The model under review builds one solid part; all positions refer to its coordinate system, in mm. A direction names the side the tool comes from. Give positions to 0.01 mm unless a question says otherwise; leave off trailing zeros. Loops run counter-clockwise (first coordinate to the right, second up) from the corner with the lowest first, then second, coordinate; pieces in that order, holes last. Notation, with made-up numbers: M 79,-5.5 L 88,-5.5 A24 ccw 88,10.5 Z; hole C 59.5,39 d3. An arc over 180 degrees is marked long. Write item = value, one per line. Start each with the question number.
1. We need section C-C on y = 1.6. Give the boundary of the cut face in (x, z).
2. Wall thickness on line 1 along Z through (x, y) = (0, -0.9); line 2 along Y through (x, z) = (5, 6); line 3 along Z through (x, y) = (-2.75, -1.3): over which ranges is each line inside the solid? List them lowest first. Write a range as from..to.
3. For faces 1 (the face through (3, -3, -3)), 2 (the face through (0.59, -2.75, 4.46)), 3 (the face through (1.73, 2.75, 7.81)), list the 3-axis set-ups (+Z, -Z, +X, -X, +Y, -Y) from which the entire face can be reached by the end or side of a thin tool; tool diameter is ignored.
4. For pin 1 (2 mm diameter, centred on y = -1, z = -7, fed in from -X); pin 2 (1.5 mm diameter, centred on x = -4.5, y = -1, fed in from -Z); pin 3 (11 mm diameter, centred on x = 0, z = 0, fed in from -Y); pin 4 (1.5 mm diameter, centred on x = -1, z = -2, fed in from -Y), all flat-tipped, find the tip position at first contact; note any pin that passes through.
5. Draft analysis for pull direction Z (two halves, no side actions). For faces 4 (the face through (-3.4, 2.5, -3.4)), 5 (the face through (-4.38, -0.04, 8.43)), 6 (the face through (3, 3, -3)), 7 (the face through (-3.233, -0.035, 1.341)), state which applies: pulls with the +Z half, pulls with the -Z half, needs draft (parallel to the pull), parting line crosses it, or undercut.
Autodesk Inventor part; units mm, degrees
ref_plane "YZ Plane" through (0, 0, 0) normal (1, 0, 0) x (0, 1, 0)
ref_plane "XZ Plane" through (0, 0, 0) normal (0, 1, 0) x (-1, 0, 0)
ref_plane "XY Plane" through (0, 0, 0) normal (0, 0, 1) x (1, 0, 0)
sketch "Эскиз1" plane through (0, 0, 0) normal (0, 1, 0) x (-1, 0, 0)
  circle A0 centre (0, 0) radius 9.5
  circle A1 centre (0, 0) radius 3.5
  circle A2 centre (0, 0) radius 8
  circle A3 centre (0, 0) radius 4.5
  dimension "d0" = 19
  dimension "d3" = 7
  dimension "d4" = 1.5
  dimension "d5" = 1
extrude "Выдавливание1" add sketch "Эскиз1" along normal mid plane 6
extrude "Выдавливание2" add sketch "Эскиз1" along normal mid plane 5 contours A2
chamfer "Фаска1" distance 0.5 angle 45 4 edges at (9.5, -3, 0) (9.5, 3, 0) (3.5, -3, 0) (3.5, 3, 0)
equation "\"d0\" = bearing_outer"
equation "\"d3\" = bearing_inner"
equation "\"d6\" = bearing_width"
equation "\"blade_radius\" = 127"
equation "\"bearing_inner\" = 7"
equation "\"bearing_outer\" = 19"
equation "\"bearing_width\" = 6"
equation "\"beam_length\" = 254"
equation "\"motor_height\" = 24"
equation "\"motor_diameter\" = 28"
equation "\"motor_blade_offset\" = 2"
equation "\"M4_nut_lock_width\" = 6.8"
equation "\"M4_screw_innerHex_cap_diam\" = 6.6"
equation "\"M4_screw_innerHex_cap_height\" = 4"
equation "\"M4_nut_lock_height\" = 5"
properties part number "Подшипник" material "Сталь, высокопрочная, низколегированная"
Final values:
q1.outline = C 0,0 d19; hole C 0,0 d7
q2.line_1 = -9.5..-3.5, 3.5..9.5
q2.line_2 = -2.5..2.5
q2.line_3 = -9.09..-2.17, 2.17..9.09
q3.face_1 = +Z, -Z, +X, -X, -Y
q3.face_2 = -Y
q3.face_3 = +Y
q4.pin_1 = -7.37
q4.pin_2 = -8.73
q4.pin_3 = -3
q4.pin_4 = through
q5.face_4 = undercut
q5.face_5 = parting line crosses it
q5.face_6 = needs draft
q5.face_7 = undercut
